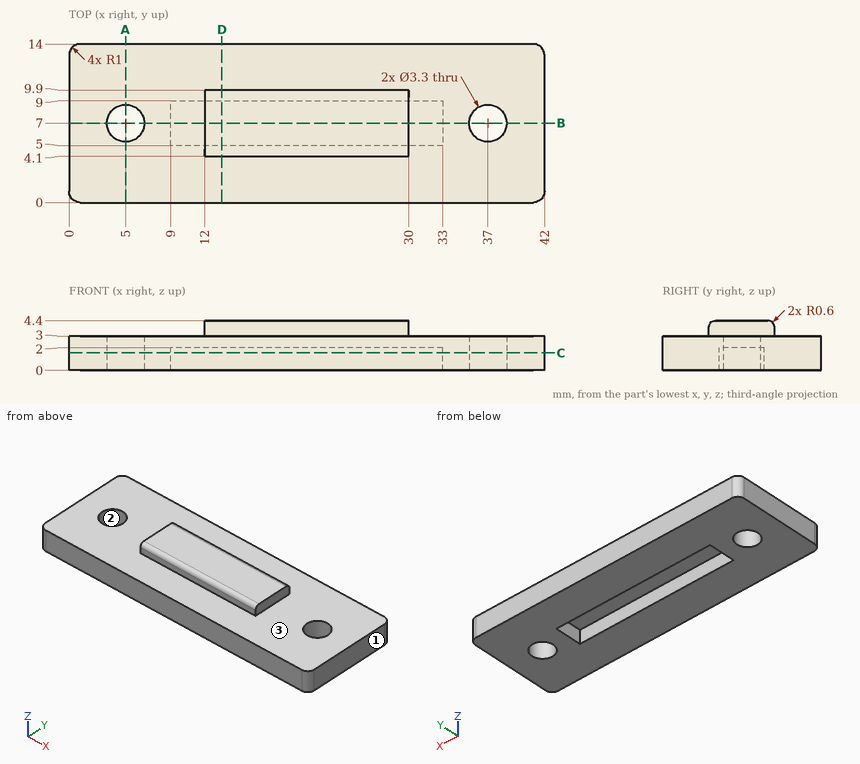
Job drawing, mm, ordinate dimensions from the low corner. One solid piece. Give positions to 0.01 mm unless a question says otherwise; leave off trailing zeros. Write each loop counter-clockwise with the first axis right and the second up, starting at its lowest first coordinate (ties: lowest second). Pieces come first, ordered by that corner, then holes. Notation, with made-up numbers: M 15.25,44 L 20.25,44 A7 cw 20.25,53 Z; hole C -36.5,-14.5 d4. An arc over 180 degrees is marked long. Put each result on its own line as item: value. Start each with the question number.
(1) Probe L1, parallel to X at y = 7, z = 1.8; L2, parallel to X at y = 7, z = 2.4; L3, parallel to Y at x = 37, z = 0.95. List the from-to ranges inside material, lowest first.
(2) Band-saw the part on C-C, the plane z = 1.55. Write the cut outline in (x, y).
(3) Band-saw the part on D-D, the plane x = 13.5. Write the cut outline in (y, z), and give its area (3 significant figures).
(4) Band-saw the part on A-A, the plane x = 5. Write the cut outline in (y, z).
(5) Band-saw the part on B-B, the plane y = 7. Write the cut outline in (x, z), and give its area (3 significant figures).
(6) Mould opens along X. For the marked faces 1, 2 and 3 say: +X half, -X half, draft (parallel to the pull), parting line (faces both ways), or undercut.
(7) Flat gauge pins, fed straight in: pin 1 Ø2 at (x, y) = (24.5, 7) entering from -Z; pin 2 Ø2.5 at (x, y) = (5, 7) entering from -Z; pin 3 Ø0.6 at (x, z) = (20.5, 3.5) entering from +Y. Where does each tip first touch, or does it go through?
Response values:
1. L1: x = 0 to 3.35, 6.65 to 9, 33 to 35.35, 38.65 to 42
1. L2: x = 0 to 3.35, 6.65 to 35.35, 38.65 to 42
1. L3: y = 0 to 5.35, 8.65 to 14
2. outline: M 0,1 A1 ccw 1,0 L 41,0 A1 ccw 42,1 L 42,13 A1 ccw 41,14 L 1,14 A1 ccw 0,13 Z; hole C 5,7 d3.3; hole M 9,5 L 33,5 L 33,9 L 9,9 Z; hole C 37,7 d3.3
3. outline: M 0,0 L 5,0 L 5,2 L 9,2 L 9,0 L 14,0 L 14,3 L 9.9,3 L 9.9,3.8 A0.6 ccw 9.3,4.4 L 4.7,4.4 A0.6 ccw 4.1,3.8 L 4.1,3 L 0,3 Z
3. area: 42.0 mm2
4. outline: M 0,0 L 5.35,0 L 5.35,3 L 0,3 Z; M 8.65,0 L 14,0 L 14,3 L 8.65,3 Z
5. outline: M 0,0 L 3.35,0 L 3.35,3 L 0,3 Z; M 6.65,0 L 9,0 L 9,2 L 33,2 L 33,0 L 35.35,0 L 35.35,3 L 30,3 L 30,4.4 L 12,4.4 L 12,3 L 6.65,3 Z; M 38.65,0 L 42,0 L 42,3 L 38.65,3 Z
5. area: 83.4 mm2
6. face 1: +X half
6. face 2: undercut
6. face 3: draft
7. pin 1: stops at z = 2
7. pin 2: passes through
7. pin 3: stops at y = 9.9
